The drawing under review shows one solid part. Ordinate dimensions are in mm from its lowest x, y, z. Round coordinates to 2 decimals unless told otherwise and drop trailing zeros. Write each loop counter-clockwise with the first axis right and the second up, starting at its lowest first coordinate (ties: lowest second). Pieces come first, ordered by that corner, then holes. Notation, with made-up numbers: (-21, 84.25) -> (12, 84.25) arc R20 cw to (12, 100.25) -> close; hole circle Ø8 at (81, 23). An arc over 180 degrees is marked (long way). Write item = value, one per line. Start each with the question number.
Item 1: For pin 1 Ø1 at (y, z) = (1.5, 24) entering from +X; pin 2 Ø0.9 at (x, y) = (12, 2) entering from +Z; pin 3 Ø1 at (x, y) = (45, 2.5) entering from +Z (1 decimal), all flat-tipped, find the tip position at first contact; note any pin that passes through.
Item 2: Add section A-A, the plane y = 2.55. State how many separate pieces and enclosed holes the cut face has, then the cut area to 3 significant figures.
Item 3: To check wall thickness, follow L1, parallel to X at y = 1, z = 39 (1 decimal); L2, parallel to X at y = 0.3, z = 15. State the ranges of each line that lie inside material, in increasing order.
Item 4: Add section B-B, the plane z = 26. State the section outline as (x, y) points.
Item 5: Add section C-C, the plane x = 58. State the section outline as (y, z) points.
Item 6: Add section D-D, the plane z = 47. State the section outline as (x, y) points.
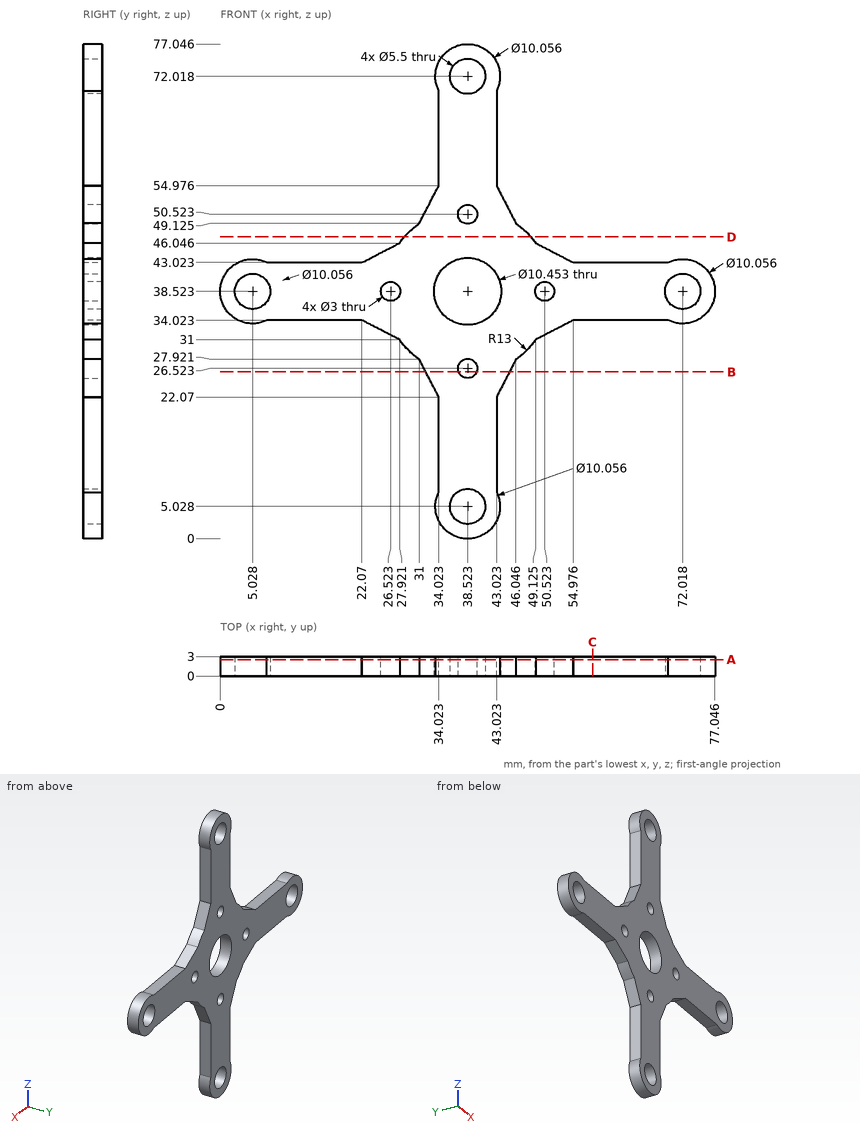
Result set:
q1.pin_1 = 44.28
q1.pin_2 = 43.02
q1.pin_3 = 52.1
q2.separate_pieces = 1
q2.enclosed_holes = 9
q2.area = 1,280 mm²
q3.L1 = 0 to 2.3, 7.7 to 25.1, 27.9 to 33.3, 43.7 to 49.1, 51.9 to 69.3, 74.7 to 77
q3.L2 = 34.02 to 43.02
q4.outline = (31.99, 0) -> (37.12, 0) -> (37.12, 3) -> (31.99, 3) -> close; (39.93, 0) -> (45.05, 0) -> (45.05, 3) -> (39.93, 3) -> close
q5.outline = (0, 34.02) -> (3, 34.02) -> (3, 43.02) -> (0, 43.02) -> close
q6.outline = (28.67, 0) -> (48.38, 0) -> (48.38, 3) -> (28.67, 3) -> close
